Model file for the job. Use its own axes, mm. Face numbers are marked on the shaded views. A direction names the side the tool comes from. Round coordinates to 2 decimals unless told otherwise and drop trailing zeros. Order: outer loops, then holes, each group sorted by start corner. A loop starts at its lowest first (then second) coordinate and runs counter-clockwise, first axis right, second up. Notation, with made-up numbers: (39, 41.5) - (48, 41.5) arc R29 cw to (48, 78.5) - close; hole circle Ø6 at (47.5, 6). An arc over 180 degrees is marked (long way). Write item = value, one per line.
Autodesk Inventor part; units mm, degrees
ref_plane "YZ Plane" through (0, 0, 0) normal (1, 0, 0) x (0, 1, 0)
ref_plane "XZ Plane" through (0, 0, 0) normal (0, 1, 0) x (-1, 0, 0)
ref_plane "XY Plane" through (0, 0, 0) normal (0, 0, 1) x (1, 0, 0)
sketch "Sketch1" plane through (0, 0, 0) normal (1, 0, 0) x (0, 1, 0)
  circle A0 centre (0, 0) radius 7.5
  circle A1 centre (0, 0) radius 9
  circle A2 centre (0, 0) radius 15
  dimension "d0" = 15
  dimension "d1" = 18
  dimension "d2" = 30
extrude "Extrusion1" add sketch "Sketch1" against normal blind 5 contours A1 | A2
extrude "Extrusion2" add sketch "Sketch1" along normal blind 10 contours A1
sketch "Sketch2" plane through (0, 0, 0) normal (1, 0, 0) x (0, 0, -1)
  point P0 (0, 0)
  point P1 (12, 0)
  dimension "d7" = 12
hole "Hole1" at (0, 0, -12) direction (-1, 0, 0) diameter 3 end through all counterbore diameter 4 counterbore depth 2
pattern_circular "Circular Pattern1" count 15 over 360 about axis through (0, 0, 0) along (-1, 0, 0) of "Hole1"
properties part number "Part2dia16"
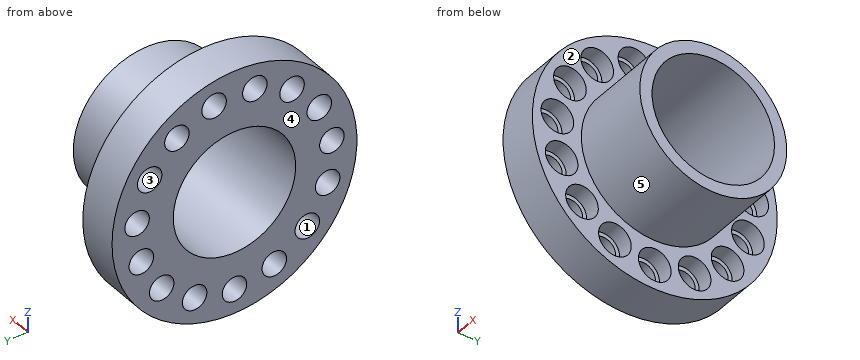
1) Flat gauge pins, fed straight in: pin 1 Ø1 at (x, y) = (4, 4) entering from -Z; pin 2 Ø1.2 at (y, z) = (-2.5, 12) entering from +X; pin 3 Ø3 at (y, z) = (-9.5, 6) entering from +X; pin 4 Ø1.5 at (x, y) = (8.5, 1) entering from +Z. Where does each tip first touch, or does it go through?
Conclusion:
pin_1 = -8.29
pin_2 = through
pin_3 = 0
pin_4 = 9
2) Cut at B-B (z = -3.5). Write the cut outline in (x, y).
Conclusion:
outline = (-5, -14.59) - (0, -14.59) - (0, -13.4) - (-2, -13.4) - (-2, -12.9) - (-5, -12.9) - close; (-5, -9.93) - (-2, -9.93) - (-2, -9.42) - (0, -9.42) - (0, -8.29) - (10, -8.29) - (10, -6.63) - (-5, -6.63) - close; (-5, 6.63) - (10, 6.63) - (10, 8.29) - (0, 8.29) - (0, 9.42) - (-2, 9.42) - (-2, 9.93) - (-5, 9.93) - close; (-5, 12.9) - (-2, 12.9) - (-2, 13.4) - (0, 13.4) - (0, 14.59) - (-5, 14.59) - close
3) Cut at D-D (x = 7.25). Write the cut outline in (y, z), and give its area (3 significant figures).
Conclusion:
outline = circle Ø18 at (0, 0); hole circle Ø15 at (0, 0)
area = 77.8 mm^2
4) Cut at A-A (y = 0). Write the cut outline in (x, z).
Conclusion:
outline = (-5, -15) - (0, -15) - (0, -14) - (-2, -14) - (-2, -13.5) - (-5, -13.5) - close; (-5, -10.5) - (-2, -10.5) - (-2, -10) - (0, -10) - (0, -9) - (10, -9) - (10, -7.5) - (-5, -7.5) - close; (-5, 7.5) - (10, 7.5) - (10, 9) - (0, 9) - (0, 15) - (-5, 15) - close
5) 3-axis set-ups, long thin cutter, end or side, ignore diameter. For the marked faces 1 and 2: which of +Z, -Z, +X, -X, +Y, -Y reach the whole face in a straight line?
Conclusion:
face_1 = +X, -X
face_2 = +X
6) Mould opens along Z. For the marked faces 3, 4 and 5 say: +Z half, -Z half, draft (parallel to the pull), parting line (faces both ways), or undercut.
Conclusion:
face_3 = undercut
face_4 = draft
face_5 = parting line
7) Wall check: line 1 along Z through (x, y) = (-2.65, 0); line 2 along Z through (x, y) = (-4, 3.25); line 3 along Y through (x, z) = (-4.5, 6.5). Give the ranges that are in metal, low to high.
Conclusion:
line_1 = -15 to -13.5, -10.5 to -7.5, 7.5 to 15
line_2 = -14.64 to -6.76, 6.76 to 10.44, 13.03 to 14.64
line_3 = -13.52 to -11.81, -8.98 to -3.74, 3.74 to 8.98, 11.81 to 13.52
